Design review of the part built by this model. Coordinates are the model's own, in mm. A direction names the side the tool comes from. Coordinates: 2 decimals unless noted, no trailing zeros. Write each loop counter-clockwise with the first axis right and the second up, starting at its lowest first coordinate (ties: lowest second). Pieces come first, ordered by that corner, then holes.
Q1. Machinability: for faces 1 (the face through (0, 18.898, -28)), 2 (the face through (-0.953, 19.098, -39.788)), which of the approach directions +Z, -Z, +X, -X, +Y, -Y give a long, thin tool a straight path to every point of the face, cutting with its end or side? Answer none if there is none.
Q2. To check wall thickness, follow probe 1 along Y at (x, z) = (3, -34); probe 2 along Y at (x, z) = (-4, -5.5); probe 3 along Y at (x, z) = (-0.75, -9.5). State the ranges of each line that lie inside material, in increasing order.
Q3. Add section A-A, the plane x = 0. Give the boundary of the cut face in (y, z), plus the area to 3 significant figures.
Q4. The part is to be moulded in two halves that separate along Z. For faces 3 (the face through (0.2, 19.1, -50.8)), 4 (the face through (0, 19.304, -25)), 5 (the face through (-0.18, -14.88, 3.3)), say which applies: +Z half, -Z half, draft (parallel to the pull), parting line (faces both ways), or undercut.
Q5. Add section B-B, the plane z = -16.5. Give the boundary of the cut face in (x, y), plus the area to 3 significant figures.
Q6. Add section D-D, the plane x = -5. Give the boundary of the cut face in (y, z), plus the area to 3 significant figures.
Q7. Clearance check with flat-ended pins moving along their axes: pin 1 Ø12 at (x, y) = (-3.5, 12.5) entering from +Z; pin 2 Ø10 at (x, z) = (-5, -7.5) entering from -Y; pin 3 Ø1 at (x, y) = (-3, -13) entering from +Z. State where each tip first meets the part, or that it passes through.
Q8. Add section C-C, the plane y = -14.5. Give the boundary of the cut face in (x, z).
from build123d import *

# Parameters (mm, degrees)
SKETCH1_R           = 15.24
BOSS_EXTRUDE1_DEPTH = 12.7
ONEHOLE_START       = -0.4064
SKETCH2_R           = 2.4892
ONEHOLE_DEPTH       = 0.4064


with BuildPart() as part:
    # Sketch1 → Boss-Extrude1 (new, symmetric)
    with BuildSketch(Plane(origin=(0, 0, 0), x_dir=(0, 0, -1), z_dir=(1, 0, 0))):
        with BuildLine():
            Line((0, 19.304), (50.8, 19.304))
            Line((50.8, 19.304), (50.8, 18.8976))
            Line((50.8, 18.8976), (3.940194188, 18.8976))
            ThreePointArc((3.940194188, 18.8976), (-1.980548611, -19.202131215), (0, 19.304))
        make_face()
        Circle(SKETCH1_R, mode=Mode.SUBTRACT)
    extrude(amount=BOSS_EXTRUDE1_DEPTH, both=True)

    # Sketch2 → OneHole (cut)
    with BuildSketch(Plane(origin=(0, 19.304, 0), x_dir=(1, 0, 0), z_dir=(0, 1, 0)).offset(ONEHOLE_START)):
        with Locations(Location((0, 42.0878, 0), (0, 0, 270))):
            Circle(SKETCH2_R)
        with BuildLine():
            Line((-12.7, 45.949031657), (-12.7, 51.435))
            Line((-12.7, 51.435), (12.7, 51.435))
            Line((12.7, 51.435), (12.7, 45.949031657))
            ThreePointArc((12.7, 45.949031657), (0, 50.8), (-12.7, 45.949031657))
        make_face()
    extrude(amount=ONEHOLE_DEPTH, mode=Mode.SUBTRACT)


solid = part.part
Here are the results:
1. face 1: -Z, +X, -X
1. face 2: +Y, -Y
2. probe 1: y = 18.9 to 19.3
2. probe 2: y = -18.5 to -14.21, 14.21 to 18.5, 18.9 to 19.3
2. probe 3: y = -16.8 to -11.92, 11.92 to 16.8, 18.9 to 19.3
3. outline: (18.9, -50.8) - (19.3, -50.8) - (19.3, -44.58) - (18.9, -44.58) - close; (18.9, -39.6) - (19.3, -39.6) - (19.3, 0) arc R19.3 ccw (long way) to (18.9, -3.94) - close; hole circle Ø30.48 at (0, 0)
3. area: 459 mm2
4. face 3: -Z half
4. face 4: draft
4. face 5: undercut
5. outline: (-12.7, -10.02) - (12.7, -10.02) - (12.7, 10.02) - (-12.7, 10.02) - close; (-12.7, 18.9) - (12.7, 18.9) - (12.7, 19.3) - (-12.7, 19.3) - close
5. area: 519 mm2
6. outline: (18.9, -50.13) - (19.3, -50.13) - (19.3, 0) arc R19.3 ccw (long way) to (18.9, -3.94) - close; hole circle Ø30.48 at (0, 0)
6. area: 460 mm2
7. pin 1: stops at z = 18.18
7. pin 2: stops at y = -19.14
7. pin 3: stops at z = 14.71
8. outline: (-12.7, -12.74) - (12.7, -12.74) - (12.7, -4.69) - (-12.7, -4.69) - close; (-12.7, 4.69) - (12.7, 4.69) - (12.7, 12.74) - (-12.7, 12.74) - close
